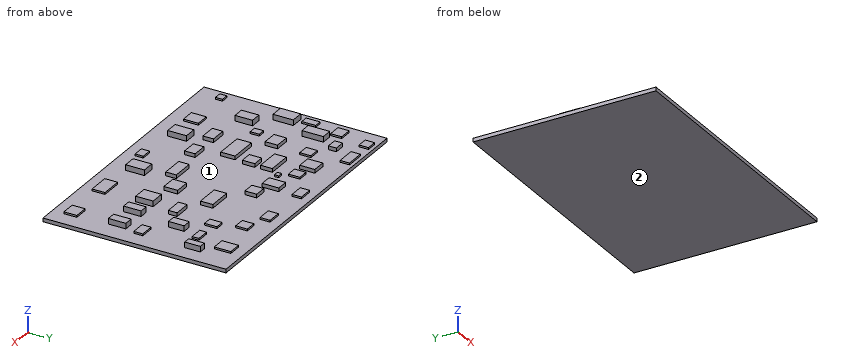
from build123d import *

# Parameters (mm, degrees)
SKETCH1_W           = 1500
SKETCH1_H           = 1000
BOSS_EXTRUDE1_DEPTH = 20
SKETCH3_W           = 130.583465718
SKETCH3_H           = 64.876118669
SKETCH3_W_2         = 151.886805153
SKETCH3_H_2         = 78.380013136
SKETCH3_W_3         = 57.534988715
SKETCH3_H_3         = 43.705768465
SKETCH3_W_4         = 74.110334533
SKETCH3_H_4         = 82.34304237
SKETCH3_W_5         = 64.654017388
SKETCH3_H_5         = 67.827502209
SKETCH3_W_6         = 64.297106784
SKETCH3_H_6         = 91.075250697
SKETCH3_W_7         = 65.482001899
SKETCH3_H_7         = 64.736542468
SKETCH3_W_8         = 82.547946155
SKETCH3_W_9         = 87.487408933
SKETCH3_H_8         = 57.683153916
SKETCH3_W_10        = 80.954123825
SKETCH3_W_11        = 120.670239475
SKETCH3_H_9         = 57.683153915
SKETCH3_W_12        = 83.987277467
SKETCH3_H_10        = 75.590177997
SKETCH3_W_13        = 128.335110014
SKETCH3_W_14        = 93.895814637
SKETCH3_H_11        = 47.906584006
BOSS_EXTRUDE3_DEPTH = 20
SKETCH4_W           = 60.505265175
SKETCH4_H           = 60.84282539
SKETCH4_W_2         = 76.713126156
SKETCH4_H_2         = 51.355111613
SKETCH4_W_3         = 57.696310853
SKETCH4_H_3         = 62.84759502
SKETCH4_W_4         = 76.226737233
SKETCH4_H_4         = 55.249628907
SKETCH4_W_5         = 61.382331515
SKETCH4_H_5         = 63.779413286
SKETCH4_W_6         = 71.885005533
SKETCH4_H_6         = 90.602849637
SKETCH4_H_7         = 37.617699495
SKETCH4_W_7         = 48.841078423
SKETCH4_H_8         = 67.384996511
SKETCH4_W_8         = 40.547503332
SKETCH4_H_9         = 49.392814631
SKETCH4_W_9         = 69.389518135
SKETCH4_W_10        = 57.1358405
SKETCH4_H_10        = 51.355111612
SKETCH4_W_11        = 101.052768507
SKETCH4_W_12        = 40.515931739
SKETCH4_H_11        = 76.411004612
SKETCH4_H_12        = 38.449288518
SKETCH4_W_13        = 76.948114593
SKETCH4_H_13        = 70.641085592
SKETCH4_W_14        = 58.340165638
SKETCH4_H_14        = 44.359686403
SKETCH4_W_15        = 74.214557021
SKETCH4_H_15        = 81.96661596
SKETCH4_W_16        = 118.257277251
SKETCH4_H_16        = 49.39281463
SKETCH4_W_17        = 27.61904506
SKETCH4_H_17        = 23.225125894
BOSS_EXTRUDE4_DEPTH = 10
SKETCH5_W           = 69.886820182
SKETCH5_H           = 110.704429614
SKETCH5_W_2         = 59.776457901
SKETCH5_H_2         = 116.965640553
SKETCH5_W_3         = 59.776457902
SKETCH5_H_3         = 95.481603563
SKETCH5_W_4         = 77.599796587
SKETCH5_W_5         = 68.98801997
SKETCH5_H_4         = 102.480565549
SKETCH5_W_6         = 68.449228886
SKETCH5_W_7         = 47.578059456
SKETCH5_H_5         = 85.302800806
SKETCH5_W_8         = 48.683008491
SKETCH5_W_9         = 37.982235028
SKETCH5_H_6         = 85.228197854
BOSS_EXTRUDE5_DEPTH = 30


with BuildPart() as part:
    # Sketch1 → Boss-Extrude1 (new body)
    with BuildSketch(Plane.XY):
        Rectangle(SKETCH1_W, SKETCH1_H)
    extrude(amount=BOSS_EXTRUDE1_DEPTH)

    # Sketch3 → Boss-Extrude3 (add)
    with BuildSketch(Plane.XY.offset(20)):
        with Locations((-251.746581796, 171.52213666)):
            Rectangle(SKETCH3_W, SKETCH3_H)
        with Locations((-279.983147389, -49.170855385)):
            Rectangle(SKETCH3_W_2, SKETCH3_H_2)
        with Locations((-542.851177133, 340.019335173)):
            Rectangle(SKETCH3_W_3, SKETCH3_H_3)
        with Locations((-317.038314656, 340.019335173)):
            Rectangle(SKETCH3_W_4, SKETCH3_H_4)
        with Locations((-218.781857631, 74.01586859)):
            Rectangle(SKETCH3_W_5, SKETCH3_H_5)
        with Locations((-68.634876688, 281.866092578)):
            Rectangle(SKETCH3_W_6, SKETCH3_H_6)
        with Locations((36.529327217, 236.328467229)):
            Rectangle(SKETCH3_W_7, SKETCH3_H_7)
        with Locations((-439.71980811, 74.01586859)):
            Rectangle(SKETCH3_W_8, SKETCH3_H_5)
        with Locations((-342.414495233, -212.465293534)):
            Rectangle(SKETCH3_W_9, SKETCH3_H_8)
        with Locations((-168.530590972, -212.465293534)):
            Rectangle(SKETCH3_W_10, SKETCH3_H_8)
        with Locations((36.529327217, -183.623716577)):
            Rectangle(SKETCH3_W_11, SKETCH3_H_9)
        with Locations((182.83360839, -109.875086681)):
            Rectangle(SKETCH3_W_12, SKETCH3_H_10)
        with Locations((197.567359377, 107.929619695)):
            Rectangle(SKETCH3_W_13, SKETCH3_H_5)
        with Locations((370.308737898, 13.972443186)):
            Rectangle(SKETCH3_W_14, SKETCH3_H_11)
    extrude(amount=BOSS_EXTRUDE3_DEPTH)

    # Sketch4 → Boss-Extrude4 (add)
    with BuildSketch(Plane.XY.offset(20)):
        with Locations((-433.57041273, 256.853926164)):
            Rectangle(SKETCH4_W, SKETCH4_H)
        with Locations((-67.526645897, 429.414434023)):
            Rectangle(SKETCH4_W_2, SKETCH4_H_2)
        with Locations((-222.402612467, 318.699136369)):
            Rectangle(SKETCH4_W_3, SKETCH4_H_3)
        with Locations((205.349756633, 416.444675835)):
            Rectangle(SKETCH4_W_4, SKETCH4_H_4)
        with Locations((342.079165749, 363.534652055)):
            Rectangle(SKETCH4_W_5, SKETCH4_H_5)
        with Locations((567.90495485, 395.424358697)):
            Rectangle(SKETCH4_W_6, SKETCH4_H_6)
        with Locations((531.962452085, 226.43251347)):
            Rectangle(SKETCH4_W_6, SKETCH4_H_7)
        with Locations((401.207804375, 226.43251347)):
            Rectangle(SKETCH4_W_7, SKETCH4_H_8)
        with Locations((-484.096796983, -54.894187693)):
            Rectangle(SKETCH4_W_8, SKETCH4_H_9)
        with Locations((-673.360372997, 287.275338859)):
            Rectangle(SKETCH4_W_9, SKETCH4_H)
        with Locations((-638.665613929, 455.091989829)):
            Rectangle(SKETCH4_W_10, SKETCH4_H_10)
        with Locations((-484.096796983, 455.091989829)):
            Rectangle(SKETCH4_W_11, SKETCH4_H_10)
        with Locations((-693.618338867, 117.106041113)):
            Rectangle(SKETCH4_W_12, SKETCH4_H_11)
        with Locations((-693.618338867, -373.3681612)):
            Rectangle(SKETCH4_W_12, SKETCH4_H_12)
        with Locations((624.860370913, -401.210769585)):
            Rectangle(SKETCH4_W_13, SKETCH4_H_13)
        with Locations((-29.170082819, -414.351469179)):
            Rectangle(SKETCH4_W_14, SKETCH4_H_14)
        with Locations((-449.070136402, -373.3681612)):
            Rectangle(SKETCH4_W_15, SKETCH4_H_15)
        with Locations((342.079165749, -401.210769585)):
            Rectangle(SKETCH4_W_16, SKETCH4_H_13)
        with Locations((624.860370913, -30.197780377)):
            Rectangle(SKETCH4_W_13, SKETCH4_H_16)
        with Locations((-168.845215562, 245.241363217)):
            Rectangle(SKETCH4_W_17, SKETCH4_H_17)
    extrude(amount=BOSS_EXTRUDE4_DEPTH)

    # Sketch5 → Boss-Extrude5 (add)
    with BuildSketch(Plane.XY.offset(20)):
        with Locations((-669.689782814, 0)):
            Rectangle(SKETCH5_W, SKETCH5_H)
        with Locations((-594.606430914, 202.16224879)):
            Rectangle(SKETCH5_W_2, SKETCH5_H_2)
        with Locations((-564.718201963, -156.448979485)):
            Rectangle(SKETCH5_W_3, SKETCH5_H_3)
        with Locations((351.696943904, -156.448979485)):
            Rectangle(SKETCH5_W_4, SKETCH5_H_3)
        with Locations((112.072703345, -351.196361502)):
            Rectangle(SKETCH5_W_5, SKETCH5_H_4)
        with Locations((-279.921964377, -351.196361502)):
            Rectangle(SKETCH5_W_6, SKETCH5_H_4)
        with Locations((503.549963007, 98.00361521)):
            Rectangle(SKETCH5_W_7, SKETCH5_H_5)
        with Locations((479.760933279, -156.448979485)):
            Rectangle(SKETCH5_W_7, SKETCH5_H_3)
        with Locations((621.042297234, -156.448979485)):
            Rectangle(SKETCH5_W_8, SKETCH5_H_3)
        with Locations((645.38380148, 266.83756344)):
            Rectangle(SKETCH5_W_9, SKETCH5_H_6)
    extrude(amount=BOSS_EXTRUDE5_DEPTH)


solid = part.part
Input: part model. Units: mm. Frame: model coordinates. Face numbers are marked on the shaded views. Round coordinates to 2 decimals unless told otherwise and drop trailing zeros.
1) Contact query for flat-ended pins moving along their axis: P1, Ø15, axis at x = 103, z = 40.5, coming from the -Y side; P2, Ø4, axis at x = 256.5, y = -70.5, coming from the +Z side; P3, Ø3, axis at y = -106.5, z = 26, coming from the -X side. Output: stop coordinate, or through.
2) Draft query along Y for the marked faces 1 and 2. Return one class per face: pulls with the +Y half, pulls with the -Y half, needs draft (parallel to the pull), parting line crosses it, or undercut.
3) Ray query, L1, parallel to X at y = -153.5, z = 23; L2, parallel to X at y = 273, z = 25; L3, parallel to Y at x = -219.5, z = 30.5. Return the intervals inside material, ascending.
Geometry says:
1. P1: stops at y = -402.44
1. P2: stops at z = 20
1. P3: stops at x = 140.84
2. face 1: undercut
2. face 2: needs draft
3. L1: x = -594.61 to -534.83, 312.9 to 390.5, 455.97 to 503.55, 596.7 to 645.38
3. L2: x = -708.06 to -638.67, -463.82 to -403.32, -100.78 to -36.49, 626.39 to 664.37
3. L3: y = -88.36 to -9.98, 40.1 to 107.93, 139.08 to 203.96
